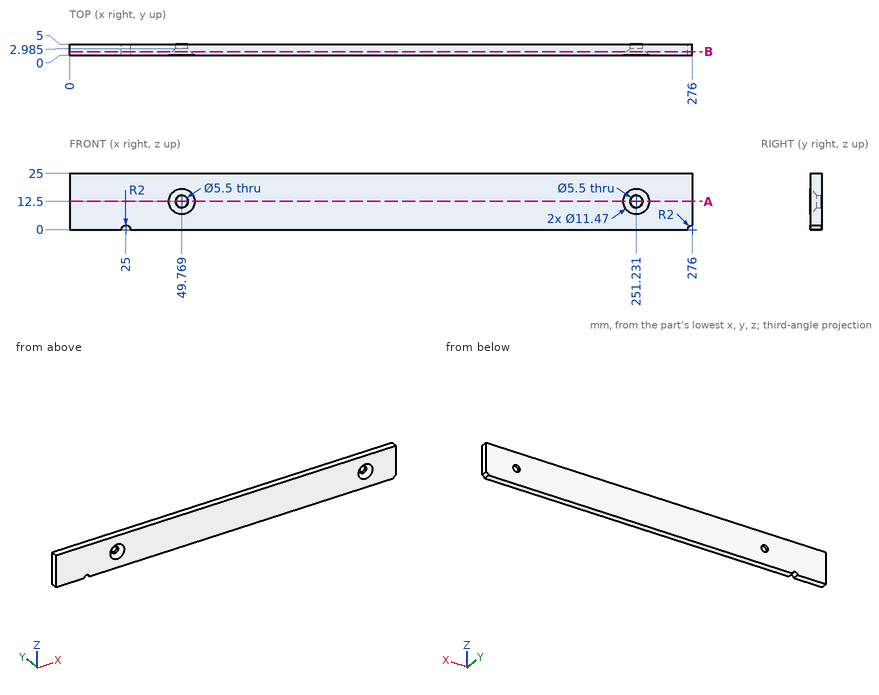
Part print with two shaded views. Sizes in mm from the minimum x, y, z corner. Coordinates: 2 decimals unless noted, no trailing zeros. Loops run counter-clockwise (first coordinate to the right, second up) from the corner with the lowest first, then second, coordinate; pieces in that order, holes last. Notation, with made-up numbers: (60.25, -31) -> (98.25, -31) arc R13 cw to (98.25, -20) -> close; hole circle Ø5 at (-35.5, -29). An arc over 180 degrees is marked (long way). Answer as a JSON object with one key per item and string values.
Q1. Probe probe 1 along X at (y, z) = (4.65, 12) (1 decimal); probe 2 along X at (y, z) = (1.8, 12) (1 decimal). List the from-to ranges inside material, lowest first.
Report:
{"probe 1": "x = 0 to 47.1, 52.5 to 248.5, 253.9 to 276", "probe 2": "x = 0 to 45.9, 53.7 to 247.3, 255.1 to 276"}
Q2. Cut at A-A (z = 12.5). List the corners of the cut face in (x, y) (1 decimal).
Report:
{"outline": "(0, 0) -> (44, 0) -> (47, 3) -> (47, 5) -> (0, 5) -> close; (52.5, 3) -> (55.5, 0) -> (245.5, 0) -> (248.5, 3) -> (248.5, 5) -> (52.5, 5) -> close; (254, 3) -> (257, 0) -> (276, 0) -> (276, 5) -> (254, 5) -> close"}
Q3. Cut at B-B (y = 1.6). List the corners of the cut face in (x, z) (1 decimal), and give its area (3 significant figures).
Report:
{"outline": "(0, 0) -> (23, 0) arc R2 cw to (27, 0) -> (274, 0) arc R2 cw to (276, 2) -> (276, 25) -> (0, 25) -> close; hole circle Ø8.3 at (49.8, 12.5); hole circle Ø8.3 at (251.2, 12.5)", "area": "6,780 mm2"}
